Geometry: final body of the model. Coordinates: model frame, mm. Face numbers are marked on the shaded views. A direction names the side the tool comes from. Give positions to 0.01 mm unless a question says otherwise; leave off trailing zeros. Loops run counter-clockwise (first coordinate to the right, second up) from the corner with the lowest first, then second, coordinate; pieces in that order, holes last.
1. Section C-C, the plane x = 1.75. Output: boundary loops of the cut face in (y, z), then the cut area to 3 significant figures.
2. Section A-A, the plane z = 2.5. Output: boundary loops of the cut face in (x, y).
3. Access query for the marked faces 1, 2 and 3. Directions: +Z, -Z, +X, -X, +Y, -Y. A direction counts if a zero-diameter tool reaches every point of the face in a straight line with its end or side. Return the directions, or none.
4. Material intervals for line 1 along Y through (x, z) = (0, 1.15) (3 decimals); line 2 along Y through (x, z) = (8.25, 0.8); line 3 along X through (y, z) = (-18.25, 0.2), sorted ascending.
5. Section B-B, the plane y = 1. Output: boundary loops of the cut face in (x, z).
6. First-contact query: P1, Ø1.2, axis at y = -0.5, z = 2.5, coming from the -X side; P2, Ø4, axis at x = 0, y = 0, coming from the +Z side (1 decimal); P3, Ø6.5, axis at x = 0.5, y = -0.5, coming from the +Z side; P4, Ø0.8, axis at y = 0, z = 2, coming from the +X side. Flat tips, straight axial feed; report the tip coordinate or a pass-through.
7. Section D-D, the plane y = -4. Output: boundary loops of the cut face in (x, z).
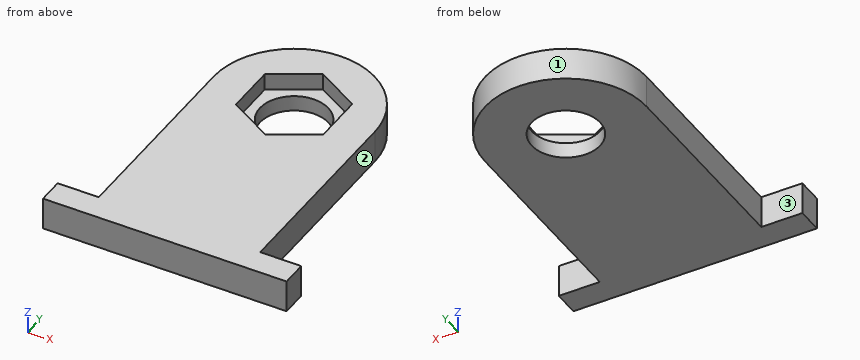
from build123d import *

# Parameters (mm, degrees)
F1_DEPTH = 2.9972
F3_DEPTH = 1.5494


with BuildPart() as f1:
    # F0 (on Top) → F1 (new body)
    with BuildSketch(Plane.XY):
        with BuildLine():
            Line((-3.175, 0), (-7.493, 0))
            Line((-7.493, 0), (-7.493, -18.6944))
            Line((-7.493, -18.6944), (-11.303, -18.6944))
            Line((-11.303, -18.6944), (-11.303, -21.082))
            Line((-11.303, -21.082), (11.303, -21.082))
            Line((11.303, -21.082), (11.303, -18.6944))
            Line((11.303, -18.6944), (7.493, -18.6944))
            Line((7.493, -18.6944), (7.493, 0))
            Line((7.493, 0), (3.175, 0))
            ThreePointArc((3.175, 0), (0, -3.175), (-3.175, 0))
        make_face()
        with BuildLine():
            ThreePointArc((7.493, 0), (0, 7.493), (-7.493, 0))
            Line((-7.493, 0), (-3.175, 0))
            ThreePointArc((-3.175, 0), (0, 3.175), (3.175, 0))
            Line((3.175, 0), (7.493, 0))
        make_face()
    extrude(amount=F1_DEPTH)

    # F2 (on face) → F3 (cut)
    with BuildSketch(Plane.XY.offset(2.9972)):
        Polygon((0, 4.692703), (-4.064, 2.346351), (-4.064, -2.346351), (0, -4.692703), (4.064, -2.346351), (4.064, 2.346351), align=None)
    extrude(amount=-F3_DEPTH, mode=Mode.SUBTRACT)


solid = f1.part
Answers below:
1. outline: (-21.08, 0) - (-2.65, 0) - (-2.65, 1.45) - (-3.68, 1.45) - (-3.68, 3) - (-21.08, 3) - close; (2.65, 0) - (7.29, 0) - (7.29, 3) - (3.68, 3) - (3.68, 1.45) - (2.65, 1.45) - close
1. area: 65.9 mm2
2. outline: (-11.3, -21.08) - (11.3, -21.08) - (11.3, -18.69) - (7.49, -18.69) - (7.49, 0) arc R7.49 ccw to (-7.49, 0) - (-7.49, -18.69) - (-11.3, -18.69) - close; hole (-4.06, -2.35) - (0, -4.69) - (4.06, -2.35) - (4.06, 2.35) - (0, 4.69) - (-4.06, 2.35) - close
3. face 1: +Z, -Z, +Y
3. face 2: +Z, -Z, +X, +Y
3. face 3: +Z, -Z, -X, +Y
4. line 1: y = -21.082 to -3.175, 3.175 to 7.493
4. line 2: y = -21.08 to -18.69
4. line 3: x = -7.49 to 7.49
5. outline: (-7.43, 0) - (-3.01, 0) - (-3.01, 1.45) - (-4.06, 1.45) - (-4.06, 3) - (-7.43, 3) - close; (3.01, 0) - (7.43, 0) - (7.43, 3) - (4.06, 3) - (4.06, 1.45) - (3.01, 1.45) - close
6. P1: stops at x = -7.49
6. P2: passes through
6. P3: stops at z = 1.45
6. P4: stops at x = 7.49
7. outline: (-7.49, 0) - (7.49, 0) - (7.49, 3) - (1.2, 3) - (1.2, 1.45) - (-1.2, 1.45) - (-1.2, 3) - (-7.49, 3) - close
